from build123d import *

# Parameters (mm, degrees)
SKETCH1_R           = 34.925
SKETCH1_R_2         = 4.318
BOSS_EXTRUDE1_DEPTH = 0.635


with BuildPart() as part:
    # Sketch1 → Boss-Extrude1 (new body)
    with BuildSketch(Plane.XY):
        with BuildLine():
            ThreePointArc((20.903132924, 39.946417348), (0, 45.085), (-20.903132924, 39.946417348))
            ThreePointArc((-20.903132924, 39.946417348), (-24.001012396, 39.224535565), (-27.060305383, 40.09556768))
            ThreePointArc((-27.060305383, 40.09556768), (-38.615101321, 38.615101321), (-40.09556768, 27.060305383))
            ThreePointArc((-40.09556768, 27.060305383), (-39.224535565, 24.001012396), (-39.946417348, 20.903132924))
            ThreePointArc((-39.946417348, 20.903132924), (-45.085, 0), (-39.946417348, -20.903132924))
            ThreePointArc((-39.946417348, -20.903132924), (-39.224535565, -24.001012396), (-40.09556768, -27.060305383))
            ThreePointArc((-40.09556768, -27.060305383), (-38.615101321, -38.615101321), (-27.060305383, -40.09556768))
            ThreePointArc((-27.060305383, -40.09556768), (-24.001012396, -39.224535565), (-20.903132924, -39.946417348))
            ThreePointArc((-20.903132924, -39.946417348), (0, -45.085), (20.903132924, -39.946417348))
            ThreePointArc((20.903132924, -39.946417348), (24.001012396, -39.224535565), (27.060305383, -40.09556768))
            ThreePointArc((27.060305383, -40.09556768), (38.615101321, -38.615101321), (40.09556768, -27.060305383))
            ThreePointArc((40.09556768, -27.060305383), (39.224535565, -24.001012396), (39.946417348, -20.903132924))
            ThreePointArc((39.946417348, -20.903132924), (45.085, 0), (39.946417348, 20.903132924))
            ThreePointArc((39.946417348, 20.903132924), (39.224535565, 24.001012396), (40.09556768, 27.060305383))
            ThreePointArc((40.09556768, 27.060305383), (38.615101321, 38.615101321), (27.060305383, 40.09556768))
            ThreePointArc((27.060305383, 40.09556768), (24.001012396, 39.224535565), (20.903132924, 39.946417348))
        make_face()
        Circle(SKETCH1_R, mode=Mode.SUBTRACT)
        with Locations((31.87990923, 31.87990923)):
            Circle(SKETCH1_R_2, mode=Mode.SUBTRACT)
        with Locations((31.87990923, -31.87990923)):
            Circle(SKETCH1_R_2, mode=Mode.SUBTRACT)
        with Locations((-31.87990923, -31.87990923)):
            Circle(SKETCH1_R_2, mode=Mode.SUBTRACT)
        with Locations((-31.87990923, 31.87990923)):
            Circle(SKETCH1_R_2, mode=Mode.SUBTRACT)
    extrude(amount=BOSS_EXTRUDE1_DEPTH)


solid = part.part
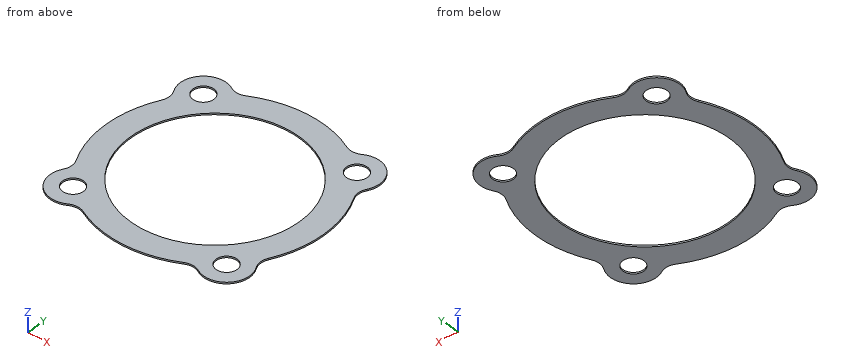
For this review, take the finished solid that the model builds, in its own axes (mm). Coordinates: 2 decimals unless noted, no trailing zeros. Loops run counter-clockwise (first coordinate to the right, second up) from the corner with the lowest first, then second, coordinate; pieces in that order, holes last. Notation, with made-up numbers: (-2, 17) - (31, 17) arc R16 ccw to (31, 23) - close; hole circle Ø8 at (-12.5, -3). An arc over 180 degrees is marked (long way). Use a Markdown table: item, result. Add a question column.
Item 1: We need section A-A (x = 0). Give the boundary of the cut face in (y, z) (3 decimals), and give its area (3 significant figures).
Item 2: We need section D-D (z = 0.4). Give the boundary of the cut face in (x, y) (3 decimals), and give its area (3 significant figures).
Item 3: Insertion check: pin 1 Ø8 at (x, y) = (11.5, -27.5) entering from +Z. The pin has a flat end and moves straight along its axis. Give the tip position at first contact, or say it passes through.
Item 4: For line 1 (Y direction, x = 0, z = 0.2) (3 decimals); line 2 (X direction, y = -35, z = 0.15); line 3 (X direction, y = -22, z = 0.6), list the stretches that pass through material, from the lowest coordinate up.
Item 5: We need section C-C (x = 32). Give the boundary of the cut face in (y, z) (3 decimals), and give its area (3 significant figures).
Results list:
| question | item | result |
|---|---|---|
| 1 | outline | (-45.085, 0) - (-34.925, 0) - (-34.925, 0.635) - (-45.085, 0.635) - close; (34.925, 0) - (45.085, 0) - (45.085, 0.635) - (34.925, 0.635) - close |
| 1 | area | 12.9 mm^2 |
| 2 | outline | (-40.096, -27.06) arc R9.525 ccw to (-27.06, -40.096) arc R6.35 cw to (-20.903, -39.946) arc R45.085 ccw to (20.903, -39.946) arc R6.35 cw to (27.06, -40.096) arc R9.525 ccw to (40.096, -27.06) arc R6.35 cw to (39.946, -20.903) arc R45.085 ccw to (39.946, 20.903) arc R6.35 cw to (40.096, 27.06) arc R9.525 ccw to (27.06, 40.096) arc R6.35 cw to (20.903, 39.946) arc R45.085 ccw to (-20.903, 39.946) arc R6.35 cw to (-27.06, 40.096) arc R9.525 ccw to (-40.096, 27.06) arc R6.35 cw to (-39.946, 20.903) arc R45.085 ccw to (-39.946, -20.903) arc R6.35 cw to start; hole circle Ø8.636 at (-31.88, -31.88); hole circle Ø8.636 at (-31.88, 31.88); hole circle Ø69.85 at (0, 0); hole circle Ø8.636 at (31.88, -31.88); hole circle Ø8.636 at (31.88, 31.88) |
| 2 | area | 2,940 mm^2 |
| 3 | pin 1 | passes through |
| 4 | line 1 | y = -45.085 to -34.925, 34.925 to 45.085 |
| 4 | line 2 | x = -40.88 to -34.86, -28.89 to 28.89, 34.86 to 40.88 |
| 4 | line 3 | x = -39.5 to -27.12, 27.12 to 39.5 |
| 5 | outline | (-41.404, 0) - (-36.196, 0) - (-36.196, 0.635) - (-41.404, 0.635) - close; (-27.564, 0) - (-13.991, 0) - (-13.991, 0.635) - (-27.564, 0.635) - close; (13.991, 0) - (27.564, 0) - (27.564, 0.635) - (13.991, 0.635) - close; (36.196, 0) - (41.404, 0) - (41.404, 0.635) - (36.196, 0.635) - close |
| 5 | area | 23.9 mm^2 |
